from build123d import *

# Parameters (mm, degrees)
SKETCH1_R           = 30
SKETCH1_R_2         = 15
BOSS_EXTRUDE1_DEPTH = 40
SKETCH2_R           = 9.5
CUT_EXTRUDE1_DEPTH  = 2.5
SKETCH3_R           = 8.25
CUT_EXTRUDE2_DEPTH  = 15
CIRPATTERN1_COUNT   = 4
SKETCH4_R           = 2
CUT_EXTRUDE3_DEPTH  = 47.904157769
CUT_EXTRUDE4_DEPTH  = 47.904157769


with BuildPart() as part:
    # Sketch1 → Boss-Extrude1 (new body)
    with BuildSketch(Plane(origin=(0, 0, 0), x_dir=(0, 0, -1), z_dir=(1, 0, 0))):
        Circle(SKETCH1_R)
        Circle(SKETCH1_R_2, mode=Mode.SUBTRACT)
    extrude(amount=BOSS_EXTRUDE1_DEPTH)

    # Sketch2 → Cut-Extrude1 (cut, symmetric)
    with BuildSketch(Plane.XY.offset(22)):
        with Locations((20, 0)):
            Circle(SKETCH2_R)
    cut_extrude1 = extrude(amount=CUT_EXTRUDE1_DEPTH, both=True, mode=Mode.SUBTRACT)

    # Sketch3 → Cut-Extrude2 (cut, symmetric)
    with BuildSketch(Plane.XY.offset(22)):
        with Locations((20, 0)):
            Circle(SKETCH3_R)
    cut_extrude2 = extrude(amount=CUT_EXTRUDE2_DEPTH, both=True, mode=Mode.SUBTRACT)

    # CirPattern1: Cut-Extrude1, Cut-Extrude2 ×4 about axis
    cirpattern1_axis = Axis((0, 0, 0), (1, 0, 0))
    add([cut_extrude1.rotate(cirpattern1_axis, i * 360 / CIRPATTERN1_COUNT) for i in range(1, CIRPATTERN1_COUNT)], mode=Mode.SUBTRACT)
    add([cut_extrude2.rotate(cirpattern1_axis, i * 360 / CIRPATTERN1_COUNT) for i in range(1, CIRPATTERN1_COUNT)], mode=Mode.SUBTRACT)


with BuildPart() as body_2:
    # Split2: the piece on the far side of the plane
    add(part.part)
    split(bisect_by=Plane(origin=(20, 0, 0), x_dir=(0, 0, 1), z_dir=(1, 0, 0)), keep=Keep.BOTTOM)


with BuildPart() as part_1:
    add(part.part)

    # Split2
    split(bisect_by=Plane(origin=(20, 0, 0), x_dir=(0, 0, 1), z_dir=(1, 0, 0)), keep=Keep.TOP)

    # Sketch4 → Cut-Extrude3 (cut, through all)
    with BuildSketch(Plane(origin=(40, 0, 0), x_dir=(0, 0, -1), z_dir=(1, 0, 0))):
        with Locations((-16.970562748, 16.970562748)):
            Circle(SKETCH4_R)
        with Locations((16.970562748, 16.970562748)):
            Circle(SKETCH4_R)
        with Locations((16.970562748, -16.970562748)):
            Circle(SKETCH4_R)
        with Locations((-16.970562748, -16.970562748)):
            Circle(SKETCH4_R)
    extrude(amount=-CUT_EXTRUDE3_DEPTH, mode=Mode.SUBTRACT)

    # Sketch5 → Cut-Extrude4 (cut, through all)
    with BuildSketch(Plane.ZY.offset(-20)):
        with BuildLine():
            ThreePointArc((-11.614095631, 9.492775288), (-11.124297731, 10.062305899), (-10.606601718, 10.606601718))
            ThreePointArc((-10.606601718, 10.606601718), (-10.062305899, 11.124297731), (-9.492775288, 11.614095631))
            Line((-9.492775288, 11.614095631), (-10.960155108, 13.081475452))
            ThreePointArc((-10.960155108, 13.081475452), (-13.081475452, 13.081475452), (-13.081475452, 10.960155108))
            Line((-13.081475452, 10.960155108), (-11.614095631, 9.492775288))
        make_face()
        with BuildLine():
            ThreePointArc((13.081475452, 10.960155108), (13.081475452, 13.081475452), (10.960155108, 13.081475452))
            Line((10.960155108, 13.081475452), (9.492775288, 11.614095631))
            ThreePointArc((9.492775288, 11.614095631), (10.606601718, 10.606601718), (11.614095631, 9.492775288))
            Line((11.614095631, 9.492775288), (13.081475452, 10.960155108))
        make_face()
        with BuildLine():
            ThreePointArc((10.960155108, -13.081475452), (13.081475452, -13.081475452), (13.081475452, -10.960155108))
            Line((13.081475452, -10.960155108), (11.614095631, -9.492775288))
            ThreePointArc((11.614095631, -9.492775288), (10.606601718, -10.606601718), (9.492775288, -11.614095631))
            Line((9.492775288, -11.614095631), (10.960155108, -13.081475452))
        make_face()
        with BuildLine():
            ThreePointArc((-13.081475452, -10.960155108), (-13.081475452, -13.081475452), (-10.960155108, -13.081475452))
            Line((-10.960155108, -13.081475452), (-9.492775288, -11.614095631))
            ThreePointArc((-9.492775288, -11.614095631), (-10.606601718, -10.606601718), (-11.614095631, -9.492775288))
            Line((-11.614095631, -9.492775288), (-13.081475452, -10.960155108))
        make_face()
    extrude(amount=-CUT_EXTRUDE4_DEPTH, mode=Mode.SUBTRACT)


solid = part_1.part
Check sheet for the modelled part. Datum: model origin and axes. Units: mm. A direction names the side the tool comes from. Give positions to 0.01 mm unless a question says otherwise; leave off trailing zeros. Order: outer loops, then holes, each group sorted by start corner. A loop starts at its lowest first (then second) coordinate and runs counter-clockwise, first axis right, second up. Notation, with made-up numbers: M 11,2 L 46,2 A22 cw 46,37 Z; hole C 50.5,7 d7. An arc over 180 degrees is marked long. Answer as CSV lines item,"result". Start each with the question number.
Item 1: Cross-section at D-D on z = -20.5. Enter the section's corners in (x, y), plus the area to 3 significant figures.
Item 2: Cross-section at C-C on x = 36.75. Enter the section's corners in (y, z).
Item 3: Tool access check on faces 1 (the face through (29.498, 0.209, -22.035)), 2 (the face through (28.25, 27.29, 0.18)), 3 (the face through (32, 15, 0)). Record the directions out of +Z, -Z, +X, -X, +Y, -Y that give a thin tool (end or side, any length) a straight path to the whole face; none if there is none.
Item 4: Mould release check, pull along Y, two halves, no side actions. Record for faces 4 (the face through (29.86, 13.1, -13.06)), 5 (the face through (40, 14, -6)): +Y half, -Y half, draft (parallel to the pull), parting line (faces both ways), or undercut.
Item 5: Cross-section at A-A on z = 0. Enter the section's corners in (x, y).
Item 6: Gauge pin test, flat ends, axial feed: P1, Ø5, axis at x = 26, y = 3, coming from the +Z side; P2, Ø3, axis at y = 15.5, z = 5.5, coming from the -X side; P3, Ø6, axis at x = 37.5, z = 19.5, coming from the +Y side. Record the tip position at first contact, or that the pin passes through.
Item 7: Thickness scan on line 1 (Y direction, x = 37.75, z = 18); line 2 (Z direction, x = 23.5, y = 12); line 3 (Z direction, x = 23.75, y = 17.5). Record the ranges inside material, lowest first. Write a range as [from, to].
Established:
1,outline,"M 20,-21.9 L 40,-21.9 L 40,21.9 L 20,21.9 L 20,9.5 A9.5 cw 20,-9.5 Z"
1,area,"734 mm^2"
2,outline,"C 0,0 d60; hole C -16.97,-16.97 d4; hole C -16.97,16.97 d4; hole M -13.08,-10.96 A1.5 ccw -10.96,-13.08 L -9.49,-11.61 A15 ccw 9.49,-11.61 L 10.96,-13.08 A1.5 ccw 13.08,-10.96 L 11.61,-9.49 A15 ccw 11.61,9.49 L 13.08,10.96 A1.5 ccw 10.96,13.08 L 9.49,11.61 A15 ccw -9.49,11.61 L -10.96,13.08 A1.5 ccw -13.08,10.96 L -11.61,9.49 A15 ccw -11.61,-9.49 Z; hole C 16.97,-16.97 d4; hole C 16.97,16.97 d4"
3,face 1,"-X"
3,face 2,"-X, +Y, -Y"
3,face 3,"+X, -X"
4,face 4,"undercut"
4,face 5,"draft"
5,outline,"M 28.25,-30 L 40,-30 L 40,-15 L 28.25,-15 L 28.25,-19.5 L 29.5,-19.5 L 29.5,-24.5 L 28.25,-24.5 Z; M 28.25,15 L 40,15 L 40,30 L 28.25,30 L 28.25,24.5 L 29.5,24.5 L 29.5,19.5 L 28.25,19.5 Z"
6,P1,"stops at z = 29.96"
6,P2,"stops at x = 24.37"
6,P3,"stops at y = 25.05"
7,line 1,"y = [-24, -18.69], [-15.26, 15.26], [18.69, 24]"
7,line 2,"z = [-27.5, -13.52], [-9.88, -9], [9, 9.88], [13.52, 27.5]"
7,line 3,"z = [-24.37, -18.9], [-15.04, -7.35], [7.35, 15.04], [18.9, 24.37]"
